```python
from build123d import *

# Parameters (mm, degrees)
SM_START               = -5
SM_BASE_FLANGE_1_DEPTH = 10
CHAMFER_1_SIZE         = 10


# Read off the part's stored shape, not the designer's step: Базовая кромка1
with BuildPart() as part:
    # Базовая кромка1 outline → Базовая кромка1 (new body)
    with BuildSketch(Plane.XY.offset(SM_START)):
        Polygon((0, 0), (-50, 0), (-50, -5), (-5, -57.5), (0, -57.5), align=None)
    extrude(amount=SM_BASE_FLANGE_1_DEPTH)

    # Фаска1
    chamfer_1_edges = [part.edges().sort_by_distance(p)[0] for p in [
        (0, 0, 0),
    ]]
    chamfer(chamfer_1_edges, length=CHAMFER_1_SIZE)


solid = part.part
```
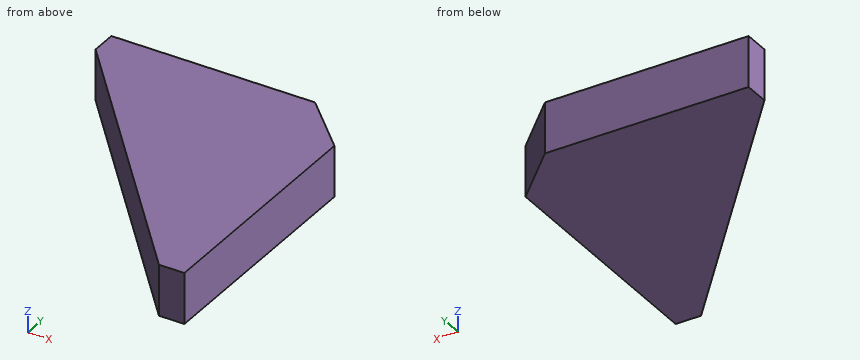
Verification items for the finished model (mm, model axes). Coordinates: 2 decimals unless noted, no trailing zeros. Loops run counter-clockwise (first coordinate to the right, second up) from the corner with the lowest first, then second, coordinate; pieces in that order, holes last. Notation, with made-up numbers: (54, -1) - (100, -1) arc R28 ccw to (100, 36) - close; hole circle Ø1 at (-14.75, 11.5). An arc over 180 degrees is marked (long way). Put each result on its own line as item: value.
Item 1: Section check A-A (z = 1). Enter the section's corners in (x, y), then the cut area to 3 significant figures.
Conclusion:
outline: (-50, -5) - (-5, -57.5) - (0, -57.5) - (0, -10) - (-10, 0) - (-50, 0) - close
area: 1,640 mm2
Item 2: Section check C-C (y = -29.5). Enter the section's corners in (x, z), then the cut area to 3 significant figures.
Conclusion:
outline: (-29, -5) - (0, -5) - (0, 5) - (-29, 5) - close
area: 290 mm2
Item 3: Scan lines: line 1 along X through (y, z) = (-5, -0.25); line 2 along X through (y, z) = (-14, -0.5); line 3 along Y through (x, z) = (-20.5, 1). Record each from-to range of solid material in increasing order.
Conclusion:
line 1: x = -50 to -5
line 2: x = -42.29 to 0
line 3: y = -39.42 to 0
Item 4: Gauge pin test, flat end, axial feed: pin 1 Ø6 at (y, z) = (-10, 1.5) entering from -X. Record the tip position at first contact, or that the pin passes through.
Conclusion:
pin 1: stops at x = -48.29
Item 5: Section check B-B (x = -33.5). Enter the section's corners in (y, z).
Conclusion:
outline: (-24.25, -5) - (0, -5) - (0, 5) - (-24.25, 5) - close
